```python
from build123d import *

# Parameters (mm, degrees)
ESQUISSE1_W             = 30
ESQUISSE1_H             = 30
BOSS_EXTRU_1_DEPTH      = 56
ESQUISSE2_W             = 17.8
ESQUISSE2_H             = 4.3
ENL_V_MAT_EXTRU_1_DEPTH = 26
ESQUISSE3_W             = 4.3
ESQUISSE3_H             = 17.8
ESQUISSE3_W_2           = 17.8
ENL_V_MAT_EXTRU_2_DEPTH = 57
ESQUISSE4_W             = 17.8
ESQUISSE4_H             = 4.3
ENL_V_MAT_EXTRU_3_DEPTH = 26


with BuildPart() as part:
    # Esquisse1 → Boss.-Extru.1 (new body)
    with BuildSketch(Plane(origin=(0, 0, 0), x_dir=(1, 0, 0), z_dir=(0, 1, 0))):
        with Locations((3.620689655, -5.615763547)):
            Rectangle(ESQUISSE1_W, ESQUISSE1_H)
    extrude(amount=BOSS_EXTRU_1_DEPTH)

    # Esquisse2 → Enlèv. mat.-Extru.1 (cut)
    with BuildSketch(Plane.XZ):
        with Locations((9.720689655, -3.284236453)):
            Rectangle(ESQUISSE2_W, ESQUISSE2_H)
    extrude(amount=-ENL_V_MAT_EXTRU_1_DEPTH, mode=Mode.SUBTRACT)

    # Esquisse3 → Enlèv. mat.-Extru.2 (cut, through all)
    with BuildSketch(Plane.XZ):
        with Locations((-5.279310345, 11.715763547)):
            Rectangle(ESQUISSE3_W, ESQUISSE3_H)
        with Locations((9.720689655, 11.715763547)):
            Rectangle(ESQUISSE3_W_2, ESQUISSE3_H)
    extrude(amount=-ENL_V_MAT_EXTRU_2_DEPTH, mode=Mode.SUBTRACT)

    # Esquisse4 → Enlèv. mat.-Extru.3 (cut)
    with BuildSketch(Plane(origin=(0, 56, 0), x_dir=(1, 0, 0), z_dir=(0, 1, 0))):
        with Locations((9.720689655, 3.284236453)):
            Rectangle(ESQUISSE4_W, ESQUISSE4_H)
    extrude(amount=-ENL_V_MAT_EXTRU_3_DEPTH, mode=Mode.SUBTRACT)


solid = part.part
```
The listing builds one solid part. Answer for the finished solid, in the listing's coordinates (mm). A direction names the side the tool comes from. Round coordinates to 2 decimals unless told otherwise and drop trailing zeros. Write each loop counter-clockwise with the first axis right and the second up, starting at its lowest first coordinate (ties: lowest second). Pieces come first, ordered by that corner, then holes. Notation, with made-up numbers: (78.5, -8.5) -> (123.5, -8.5) arc R10 ccw to (123.5, 0.5) -> close; hole circle Ø8 at (29, 66.25). An arc over 180 degrees is marked (long way). Use CSV: the item, a comma, the result in double quotes. Start each with the question number.
(1) Section A-A on z = 11 is taken. Give the vertices of the cut face in (x, y), then the cut area to 3 significant figures.
(2) Section D-D on x = -5.75 is taken. Give the vertices of the cut face in (y, z), then the cut area to 3 significant figures.
(3) Which of the six approach directions +Z, -Z, +X, -X, +Y, -Y give full straight-line access (tool end or side, diameter ignored) to faces 1 (the face through (-5, 28, 2.816)), 2 (the face through (10, 28, 2.816)), 3 (the face through (10, 30, -3)), 4 (the face through (10, 26, -3))?
(4) Consider L1, parallel to Z at x = 10, y = 41; L2, parallel to X at y = 24, z = 3; L3, parallel to X at y = 52, z = -3.25. Determine where each line is inside the solid, lowest interval first. Write a range as from..to.
(5) Section B-B on x = 6.5 is taken. Give the vertices of the cut face in (y, z).
(6) Section C-C on y = 29 is taken. Give the vertices of the cut face in (x, z), then the cut area to 3 significant figures.
(7) The mould has two halves that part along Z. Classify faces 5 (the face through (18.621, 28, -3)), 6 (the face through (10, 43, -1.134)), 7 (the face through (-9, 28, 20.616)), 8 (the face through (3, 28, -9.384)): released by +Z, released by -Z, zero draft, split by the parting line, or undercut.
(8) Each of these flat-tipped pins is pushed along its axis until it touches: pin 1 (1.3 mm diameter, centred on x = -5, y = 38.5, fed in from +Z); pin 2 (9 mm diameter, centred on y = 37.5, z = 11.5, fed in from +X); pin 3 (3.5 mm diameter, centred on x = 10, z = -3.5, fed in from +Y). Where does it stop, or does it pass through?
A:
1,outline,"(-11.38, 0) -> (-7.43, 0) -> (-7.43, 56) -> (-11.38, 56) -> close; (-3.13, 0) -> (0.82, 0) -> (0.82, 56) -> (-3.13, 56) -> close"
1,area,"442 mm²"
2,outline,"(0, -9.38) -> (56, -9.38) -> (56, 2.82) -> (0, 2.82) -> close"
2,area,"683 mm²"
3,face 1,"+Z, +Y, -Y"
3,face 2,"+Z, +X, +Y, -Y"
3,face 3,"+X, +Y"
3,face 4,"+X, -Y"
4,L1,"z = -9.38..-5.43, -1.13..2.82"
4,L2,"x = -11.38..-7.43, -3.13..0.82"
4,L3,"x = -11.38..0.82"
5,outline,"(0, -9.38) -> (56, -9.38) -> (56, -5.43) -> (30, -5.43) -> (30, -1.13) -> (56, -1.13) -> (56, 2.82) -> (0, 2.82) -> (0, -1.13) -> (26, -1.13) -> (26, -5.43) -> (0, -5.43) -> close"
6,outline,"(-11.38, -9.38) -> (18.62, -9.38) -> (18.62, 2.82) -> (0.82, 2.82) -> (0.82, 20.62) -> (-3.13, 20.62) -> (-3.13, 2.82) -> (-7.43, 2.82) -> (-7.43, 20.62) -> (-11.38, 20.62) -> close"
6,area,"507 mm²"
7,face 5,"zero draft"
7,face 6,"undercut"
7,face 7,"released by +Z"
7,face 8,"released by -Z"
8,pin 1,"stops at z = 2.82"
8,pin 2,"stops at x = 0.82"
8,pin 3,"stops at y = 30"
